Check sheet for the modelled part. Datum: model origin and axes. Units: mm. A direction names the side the tool comes from. Give positions to 0.01 mm unless a question says otherwise; leave off trailing zeros. Write each loop counter-clockwise with the first axis right and the second up, starting at its lowest first coordinate (ties: lowest second). Pieces come first, ordered by that corner, then holes. Notation, with made-up numbers: (-32.5, -38.75) -> (-0.5, -38.75) arc R27 ccw to (-0.5, -20.75) -> close; hole circle Ø3 at (8.25, 22.25). An arc over 180 degrees is marked (long way). Return JSON: item names as keys, results as strings.
Autodesk Inventor part; units mm, degrees
ref_plane "Plan de construction1" through (0, 0, 0) normal (0, 0.5, -0.8660254) x (1, 0, 0)
ref_plane "Plan de construction2" through (0, 0, 15) normal (0, 0, 1) x (1, 0, 0)
ref_plane "Plan de construction3" through (-37, -25.9808, 15) normal (1, 0, 0) x (0, 0, -1)
ref_plane "Plan de construction1" through (0, 0, 0) normal (0, 0.5, -0.8660254) x (1, 0, 0)
sketch "Esquisse1" plane through (0, 0, 0) normal (0, 0.5, -0.8660254) x (1, 0, 0)
  line L0 (-40, 0) -> (-40, -30)
  line L1 (-40, -30) -> (-37, -30)
  line L2 (-40, -30) -> (-37, -30)
  line L3 (-37, -30) -> (-37, 30)
  line L4 (-37, 30) -> (-40, 30)
  line L5 (-40, 30) -> (-40, -30)
  point P0 (0, 0)
  point P1 (-37, 0)
  point P2 (-37, -30)
  dimension "d2" = 30
  dimension "d3" = 3
  dimension "d4" = 60
  dimension "d49" = 37
  dimension "d50" = 40
extrude "Extrusion1" add sketch "Esquisse1" along normal blind 70
ref_plane "Plan de construction2" through (0, 0, 15) normal (0, 0, 1) x (1, 0, 0)
sketch "Esquisse2" plane through (0, 0, 15) normal (0, 0, 1) x (1, 0, 0)
  line L0 (-40, -25.9808) -> (-40, 25.9808)
  line L1 (-37, 25.9808) -> (-37, -25.9808)
  line L2 (-40, 25.9808) -> (-37, 25.9808)
  line L3 (-37, -25.9808) -> (-40, -25.9808)
  line L4 (-37, 60.9808) -> (-37, 9.0192)
  line L5 (-40, 25.9808) -> (-37, 25.9808)
  line L6 (-37, 25.9808) -> (-37, 35.9808)
  line L7 (-37, 35.9808) -> (-40, 35.9808)
  line L8 (-40, 35.9808) -> (-40, 25.9808)
  point P0 (0, 0)
  point P1 (37, 25.9808)
  dimension "d46" = 10
extrude "Extrusion2" add sketch "Esquisse2" against normal blind 30 contours L0 L2 L1 L3
ref_plane "Plan de construction3" through (-37, -25.9808, 15) normal (1, 0, 0) x (0, 0, -1)
sketch "Esquisse3" plane through (-37, -25.9808, 15) normal (1, 0, 0) x (0, 0, -1)
  line L0 (0, 0) -> (0, 20)
  line L1 (0, 51.9615) -> (0, 0)
  line L2 (0, 20) -> (-5, 20)
  line L3 (-5, 20) -> (-5, 25)
  line L4 (-5, 25) -> (0, 25)
  point P0 (15, 25.9808)
  dimension "d16" = 20
  dimension "d17" = 5
extrude "Extrusion3" add sketch "Esquisse3" against normal up to surface (3 mm away)
sketch "Esquisse13" plane through (0, 35, -60.6218) normal (0, 0.5, -0.8660254) x (-1, 0, 0)
  line L0 (37, 30) -> (37, -30)
  line L1 (37, 0) -> (37, 20)
  line L2 (37, 20) -> (40, 20)
  line L3 (40, -30) -> (40, 30)
  line L4 (40, 20) -> (40, 23)
  line L5 (40, 23) -> (37, 23)
  line L6 (37, 23) -> (37, 17)
  line L7 (37, 17) -> (40, 17)
  line L8 (40, 17) -> (40, 20)
  line L9 (37, 0) -> (37, -20)
  line L10 (37, -20) -> (40, -20)
  line L11 (40, -20) -> (40, -17)
  line L12 (40, -17) -> (37, -17)
  line L13 (37, -17) -> (37, -23)
  line L14 (37, -23) -> (40, -23)
  line L15 (40, -23) -> (40, -20)
  point P0 (0, 0)
  point P1 (37, 23)
  point P2 (37, 17)
  point P3 (40, 17)
  dimension "d53" = 20
  dimension "d54" = 3
  dimension "d55" = 6
  dimension "d56" = 20
  dimension "d57" = 3
  dimension "d58" = 6
extrude "Extrusion12" add sketch "Esquisse13" along normal blind 5 contours L5 L3 L2 L0 | L2 L3 L7 L0 | L12 L3 L10 L0 | L10 L3 L14 L0
sketch "Esquisse14" plane through (-37, -25.9808, 15) normal (1, 0, 0) x (0, 0, -1)
  line L0 (11.2627, 44.9296) -> (54.564, 69.9296)
  line L1 (11.2627, 44.9296) -> (61.2627, 44.9296) construction
  arc A0 (59.564, 61.2694) -> (54.564, 69.9296) centre (57.064, 65.5995) ccw
  line L2 (59.564, 61.2694) -> (16.2401, 36.3085)
  line L3 (26.3922, 19.4858) -> (76.3922, 19.4858) construction
  line L4 (11.2627, 44.9296) -> (9.7627, 47.5277)
  line L5 (9.7627, 47.5277) -> (53.064, 72.5277)
  line L6 (59.564, 61.2694) -> (61.064, 58.6713)
  line L7 (61.064, 58.6713) -> (17.7627, 33.6713)
  line L8 (17.7627, 33.6713) -> (22.7627, 25.011)
  line L9 (17.7627, 33.6713) -> (27.7627, 33.6713) construction
  line L10 (22.7627, 25.011) -> (66.064, 50.011)
  line L11 (17.7627, 33.6713) -> (22.7627, 25.011)
  arc A1 (17.7627, 33.6713) -> (22.7627, 25.011) centre (20.2627, 29.3412) ccw
  line L12 (22.7627, 25.011) -> (24.2627, 22.413)
  line L13 (24.2627, 22.413) -> (67.564, 47.413)
  arc A2 (16.2401, 36.3085) -> (24.2853, 22.3738) centre (20.2627, 29.3412) ccw
  arc A3 (61.064, 58.6713) -> (53.064, 72.5277) centre (57.064, 65.5995) ccw
  line L14 (67.564, 47.413) -> (72.564, 38.7527)
  line L15 (67.564, 47.413) -> (77.564, 47.413) construction
  line L16 (72.564, 38.7527) -> (29.2627, 13.7527)
  line L17 (29.2627, 13.7527) -> (30.7627, 11.1546)
  line L18 (30.7627, 11.1546) -> (74.064, 36.1546)
  arc A4 (72.564, 38.7527) -> (67.564, 47.413) centre (70.064, 43.0828) ccw
  arc A5 (74.064, 36.1546) -> (66.064, 50.011) centre (70.064, 43.0828) ccw
  line L19 (16.2401, 36.3085) -> (17.7627, 33.6713)
  line L20 (22.7627, 25.011) -> (24.2853, 22.3738)
  line L21 (59.564, 61.2694) -> (61.064, 58.6713)
  dimension "d61" = 50
  dimension "d62" = 30
  dimension "d63" = 10
  dimension "d64" = 5
  dimension "d71" = 3
  dimension "d72" = 3
  dimension "d75" = 10
  dimension "d76" = 60
  dimension "d78" = 90
  dimension "d79" = 3
  dimension "d80" = 10
  dimension "d81" = 60
  dimension "d82" = 50
  dimension "d83" = 90
  dimension "d84" = 3
  dimension "d85" = 5
extrude "Extrusion13" add sketch "Esquisse14" against normal blind 5 contours L4 L5 A3 L6 A0 L0 | L6 L7 L19 L2 | L19 A1 L12 L20 A2 | L12 L10 A5 L18 L17 L16 A4 L13
properties part number "autour hélice autre côté"
(1) Thickness scan on L1, parallel to X at y = 43, z = -40; L2, parallel to Y at x = -40.95, z = -56; L3, parallel to Y at x = -40.55, z = -52.5. Record the ranges inside material, lowest first.
Reply:
{"L1": "-40 to -37", "L2": "8.4 to 11.87, 22.01 to 25.05", "L3": "6.38 to 9.85, 21.4 to 24.68"}
(2) Cross-section at D-D on z = -29. Enter the section's corners in (x, y).
Reply:
{"outline": "(-42, -7.18) -> (-40, -7.18) -> (-40, -17.9) -> (-37, -17.9) -> (-37, 51.38) -> (-40, 51.38) -> (-40, 41.31) -> (-42, 41.31) -> (-42, 37.85) -> (-40, 37.85) -> (-40, 26.32) -> (-42, 26.32) -> (-42, 22.84) -> (-40, 22.84) -> (-40, 11.29) -> (-42, 11.29) -> (-42, 7.83) -> (-40, 7.83) -> (-40, -3.72) -> (-42, -3.72) -> close"}
(3) Release check for a two-part mould opening along Z. For faces 4 (the flat face through (-40.986, -13.509, -15.002)), 5 (the flat face through (-40.986, 22.983, -23.205)), 6 (the flat face through (-40.99, -2.5, -37.11)) record: pulls with the +Z half, pulls with the -Z half, needs draft (parallel to the pull), parting line crosses it, or undercut.
Reply:
{"face 4": "pulls with the +Z half", "face 5": "undercut", "face 6": "pulls with the -Z half"}
(4) Cross-section at B-B on z = -4. Enter the section's corners in (x, y), then the cut area to 3 significant figures.
Reply:
{"outline": "(-42, -4.59) -> (-40, -4.59) -> (-40, -25.98) -> (-37, -25.98) -> (-37, 36.95) -> (-40, 36.95) -> (-40, 26.88) -> (-42, 26.88) -> (-42, 23.42) -> (-40, 23.42) -> (-40, 11.92) -> (-42, 11.92) -> (-42, 8.4) -> (-40, 8.4) -> (-40, -1.48) -> (-42, -1.48) -> close", "area": "209 mm^2"}
(5) Set-up check for faces 1 (the flat face through (-40.986, 20.23, 4.477)), 2 (the flat face through (-38.521, 56.151, -51.257)), 3 (the cylindrical face through (-40.986, 0.956, -0.879)): record each of +Z, -Z, +X, -X, +Y, -Y from which the full face is reachable in a straight line by a thin tool's end or side.
Reply:
{"face 1": "+Z, -X, -Y", "face 2": "+X, -X, +Y", "face 3": "-X"}
(6) Cross-section at A-A on y = -8.5. Enter the section's corners in (x, z).
Reply:
{"outline": "(-42, -26.72) -> (-40, -26.72) -> (-40, -45.28) -> (-37, -45.28) -> (-37, 15) -> (-40, 15) -> (-40, -20.72) -> (-42, -20.72) -> close"}
(7) Cross-section at C-C on x = -38.8. Enter the section's corners in (y, z).
Reply:
{"outline": "(-25.98, -15) -> (9.02, -75.62) -> (15.08, -72.12) -> (17.58, -76.45) -> (22.78, -73.45) -> (20.28, -69.12) -> (49.72, -52.12) -> (52.22, -56.45) -> (57.42, -53.45) -> (54.92, -49.12) -> (60.98, -45.62) -> (25.98, 15) -> (-0.98, 15) -> (-0.98, 20) -> (-5.98, 20) -> (-5.98, 15) -> (-25.98, 15) -> close"}
(8) Depth check by flat-ended pin: pin 1 Ø2 at (x, z) = (-39.5, -6.5) entering from +Y; pin 2 Ø2 at (x, z) = (-37.5, -40) entering from -Y; pin 3 Ø2.5 at (x, z) = (-39, 18) entering from -Y. Enter the tip coordinate at first touch or a pass-through.
Reply:
{"pin 1": "y = 38.97", "pin 2": "y = -12.12", "pin 3": "y = -5.98"}
